Print and shaded views of the part. All mm, measured from the part's lowest x, y and z. Round coordinates to 2 decimals unless told otherwise and drop trailing zeros. Order: outer loops, then holes, each group sorted by start corner. A loop starts at its lowest first (then second) coordinate and runs counter-clockwise, first axis right, second up. Notation, with made-up numbers: M 17.25,81 L 40.25,81 A18 cw 40.25,107 Z; hole C -33,29.5 d9. An arc over 180 degrees is marked long. Use CSV: the item, a comma, the result in double quotes.
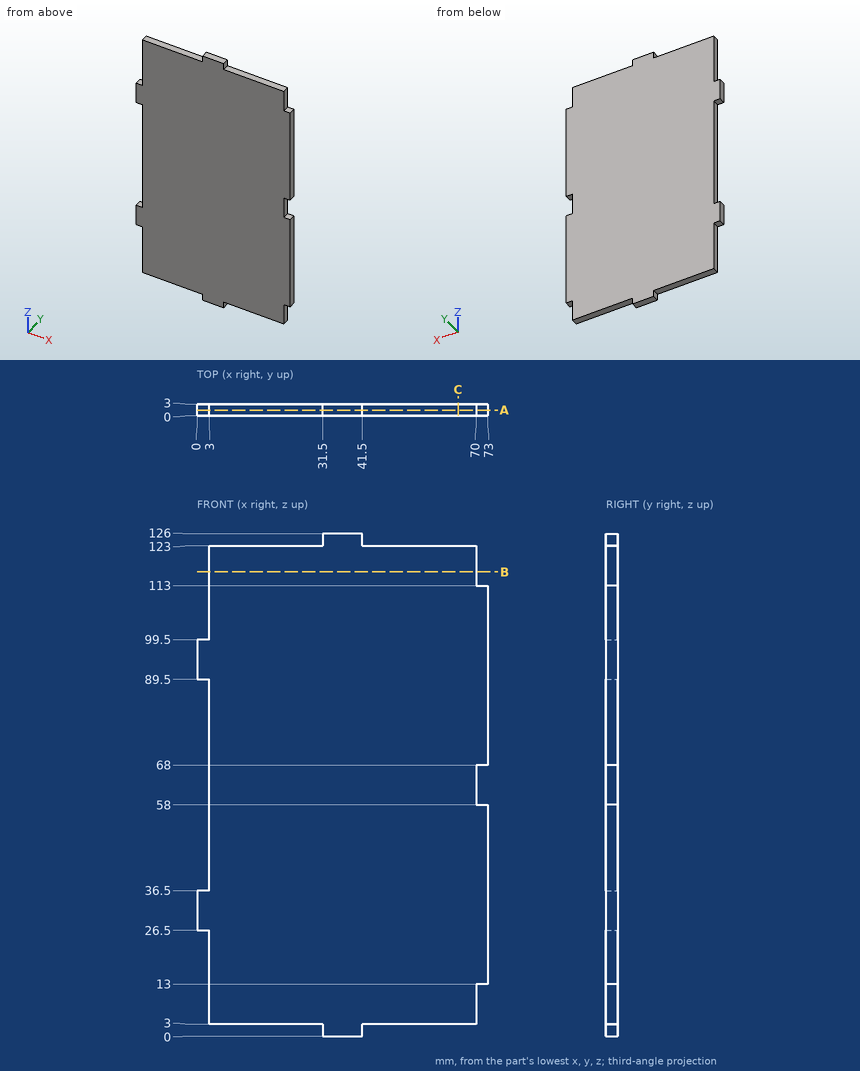
(1) Cut at C-C, the plane x = 65.5. Give the cut face in (y, z), and give its area (3 significant figures).
Answer block:
outline,"M 0,3 L 3,3 L 3,123 L 0,123 Z"
area,"360 mm²"
(2) Cut at A-A, the plane y = 1.45. Give the cut face in (x, z).
Answer block:
outline,"M 0,26.5 L 3,26.5 L 3,3 L 31.5,3 L 31.5,0 L 41.5,0 L 41.5,3 L 70,3 L 70,13 L 73,13 L 73,58 L 70,58 L 70,68 L 73,68 L 73,113 L 70,113 L 70,123 L 41.5,123 L 41.5,126 L 31.5,126 L 31.5,123 L 3,123 L 3,99.5 L 0,99.5 L 0,89.5 L 3,89.5 L 3,36.5 L 0,36.5 Z"
(3) Drop flat-ended pins along their axis: pin 1 (1 mm diameter, centred on y = 2.5, z = 81.5, fed in from -X); pin 2 (1.5 mm diameter, centred on x = 71.5, y = 1, fed in from -Z); pin 3 (1.5 mm diameter, centred on x = 1, y = 1.5, fed in from +Z). Give the stop position or say it passes through.
Answer block:
pin 1,"stops at x = 3"
pin 2,"stops at z = 13"
pin 3,"stops at z = 99.5"
(4) Cut at B-B, the plane z = 116.5. Give the cut face in (x, y).
Answer block:
outline,"M 3,0 L 70,0 L 70,3 L 3,3 Z"
(5) Wall check: line 1 (X direction, y = 2.1, z = 86); line 2 (Z direction, x = 50, y = 2.9); line 3 (X direction, y = 0.8, z = 61). Give the ranges that are in metal, low to high. Write a range as from..to.
Answer block:
line 1,"x = 3..73"
line 2,"z = 3..123"
line 3,"x = 3..70"
